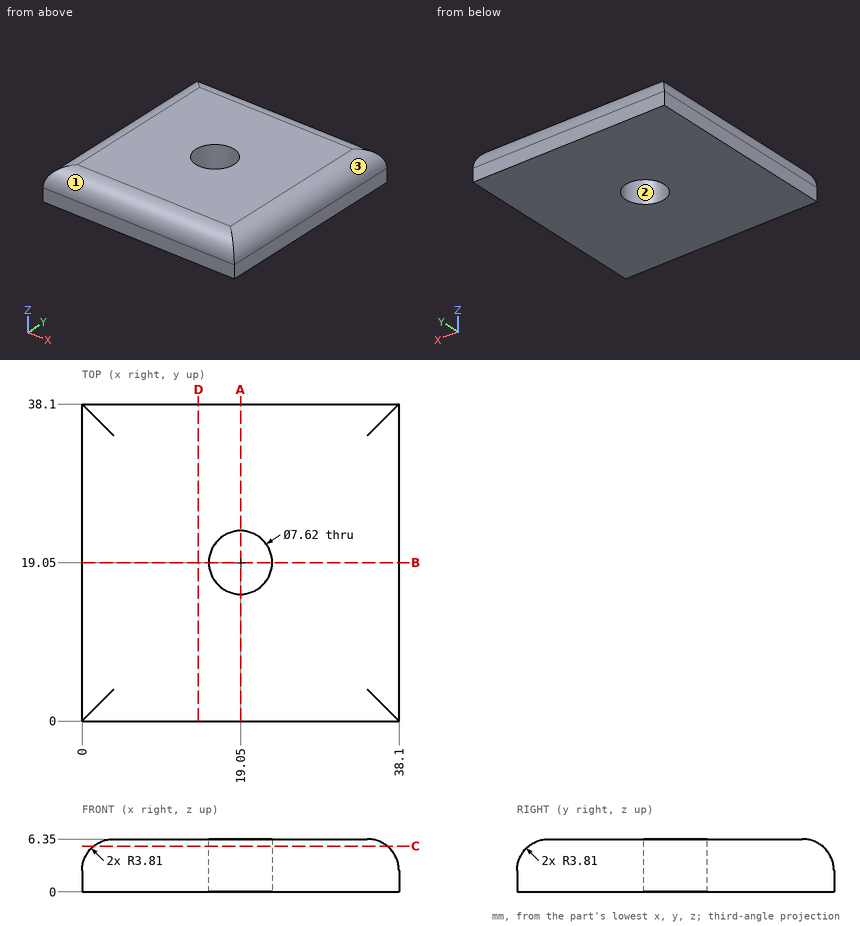
Design review of the part shown in the three views and the two pictorial views. Dimensions are in mm from the part's minimum x, y and z. Coordinates: 2 decimals unless noted, no trailing zeros. Loops run counter-clockwise (first coordinate to the right, second up) from the corner with the lowest first, then second, coordinate; pieces in that order, holes last. Notation, with made-up numbers: (57.25, 21) - (93.25, 21) arc R17 ccw to (93.25, 39) - close; hole circle Ø5 at (-35.75, 39). An arc over 180 degrees is marked (long way). Use a Markdown table: item, result. Add a question column.
Item 1: We need section C-C (z = 5.5). Give the boundary of the cut face in (x, y).
Item 2: We need section D-D (x = 14). Give the boundary of the cut face in (y, z), and give its area (3 significant figures).
Item 3: We need section A-A (x = 19.05). Give the boundary of the cut face in (y, z), and give its area (3 significant figures).
Item 4: Mouldability with a two-part tool opening along X and no side actions: class the marked faces 1, 2 and 3 as pulls with the +X half, pulls with the -X half, needs draft (parallel to the pull), parting line crosses it, or undercut.
Item 5: For line 1 (Y direction, x = 19.05, z = 1.75); line 2 (Y direction, x = 19.05, z = 4.75); line 3 (X direction, y = 20, z = 2.5), list the stretches that pass through material, from the lowest coordinate up.
Results list:
| question | item | result |
|---|---|---|
| 1 | outline | (1.41, 1.41) - (36.69, 1.41) - (36.69, 36.69) - (1.41, 36.69) - close; hole circle Ø7.62 at (19.05, 19.05) |
| 2 | outline | (0, 0) - (38.1, 0) - (38.1, 2.54) arc R3.81 ccw to (34.29, 6.35) - (3.81, 6.35) arc R3.81 ccw to (0, 2.54) - close |
| 2 | area | 236 mm^2 |
| 3 | outline | (0, 0) - (15.24, 0) - (15.24, 6.35) - (3.81, 6.35) arc R3.81 ccw to (0, 2.54) - close; (22.86, 0) - (38.1, 0) - (38.1, 2.54) arc R3.81 ccw to (34.29, 6.35) - (22.86, 6.35) - close |
| 3 | area | 187 mm^2 |
| 4 | face 1 | needs draft |
| 4 | face 2 | undercut |
| 4 | face 3 | pulls with the +X half |
| 5 | line 1 | y = 0 to 15.24, 22.86 to 38.1 |
| 5 | line 2 | y = 0.71 to 15.24, 22.86 to 37.39 |
| 5 | line 3 | x = 0 to 15.36, 22.74 to 38.1 |
